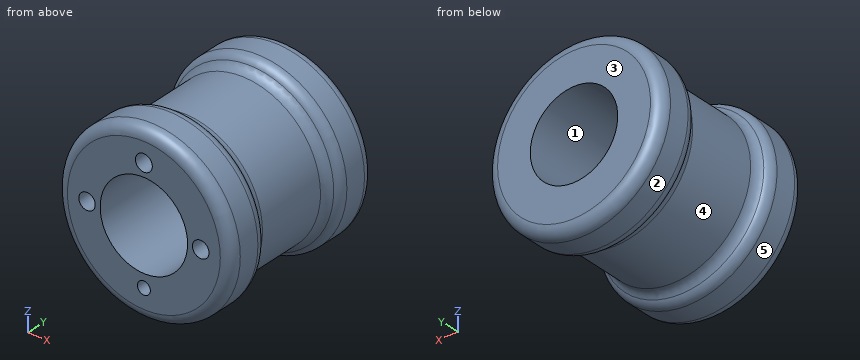
```python
from build123d import *

# Parameters (mm, degrees)
F0_R          = 12.7
F0_R_2        = 6.35
F1_DEPTH      = 25.4
F2_R          = 3.3757627259
F3_DEPTH      = 6.35
F4_R          = 12.7
F4_R_2        = 11.1125
F5_DEPTH      = 12.7
F6_R          = 4.2817922897
F7_DEPTH      = 25.4
F8_R          = 1.2247027219
F8_R_2        = 1.2053090412
F8_R_3        = 0.9363200651
F8_R_4        = 1.1938
F9_DEPTH      = 3.175
F10_S7_R      = 11.1125
F10_T8_DEPTH  = 21
F10_S13_R     = 11.1125
F10_T14_DEPTH = 21
F11_R         = 1.6002


# Not quite as in the source:
# - a fillet or chamfer that OpenCascade refuses, or shapes differently, is made with other operations: its cross-section is extruded or revolved along the edge and cut away or added


with BuildPart() as f1:
    # F0 (on Front) → F1 (new body)
    with BuildSketch(Plane.XZ):
        Circle(F0_R)
        Circle(F0_R_2, mode=Mode.SUBTRACT)
    extrude(amount=F1_DEPTH)

    # F4 (on face) → F5 (cut)
    with BuildSketch(Plane.XZ.offset(6.35)):
        Circle(F4_R)
        Circle(F4_R_2, mode=Mode.SUBTRACT)
    extrude(amount=F5_DEPTH, mode=Mode.SUBTRACT)

    # F8 (on face) → F9 (cut)
    with BuildSketch(Plane.XZ.offset(25.4)):
        with Locations((0, 8.255)):
            Circle(F8_R)
        with Locations((8.255, 0)):
            Circle(F8_R_2)
        with Locations((0, -8.255)):
            Circle(F8_R_3)
        with Locations((-8.255, 0)):
            Circle(F8_R_4)
    extrude(amount=-F9_DEPTH, mode=Mode.SUBTRACT)

    # F10: fillet of radius 1.6002 on 4 edges, made by hand

    # F10_s1 → F10_t2 (revolve, cut)
    with BuildSketch(Plane.XY):
        with BuildLine():
            ThreePointArc((11.0998, -25.4), (12.2313122713, -24.9313122713), (12.7, -23.7998))
            Line((12.7, -23.7998), (12.7, -25.4))
            Line((12.7, -25.4), (11.0998, -25.4))
        make_face()
    revolve(axis=Axis((0, -25.4, 0), (0, -1, 0)), mode=Mode.SUBTRACT)


with BuildPart() as f3:
    # F2 (on Front) → F3 (new body)
    with BuildSketch(Plane.XZ):
        Circle(F2_R)
    extrude(amount=F3_DEPTH)

    # F6 (on face) → F7 (cut)
    with BuildSketch(Plane.XZ.offset(6.35)):
        Circle(F6_R)
    extrude(amount=-F7_DEPTH, mode=Mode.SUBTRACT)


with BuildPart() as f10_tool4:
    # F10_s5 → F10_t6 (revolve)
    with BuildSketch(Plane.XY):
        with BuildLine():
            ThreePointArc((11.0998, -19.05), (12.2313122713, -19.5186877287), (12.7, -20.6502))
            Line((12.7, -20.6502), (12.7, -19.05))
            Line((12.7, -19.05), (11.0998, -19.05))
        make_face()
    revolve(axis=Axis((0, -19.05, 0), (0, -1, 0)))

    # F10_s7 → F10_t8 (cut, symmetric)
    with BuildSketch(Plane.XZ.offset(20.4)):
        Circle(F10_S7_R)
    extrude(amount=F10_T8_DEPTH, both=True, mode=Mode.SUBTRACT)


with BuildPart() as f1_1:
    add(f1.part)

    # F10_t3: cut F10_tool4
    add(f10_tool4.part, mode=Mode.SUBTRACT)


with BuildPart() as f10_tool10:
    # F10_s11 → F10_t12 (revolve)
    with BuildSketch(Plane.XY):
        with BuildLine():
            ThreePointArc((12.7, -4.7498), (12.2313122713, -5.8813122713), (11.0998, -6.35))
            Line((11.0998, -6.35), (12.7, -6.35))
            Line((12.7, -6.35), (12.7, -4.7498))
        make_face()
    revolve(axis=Axis((0, -6.35, 0), (0, -1, 0)))

    # F10_s13 → F10_t14 (cut, symmetric)
    with BuildSketch(Plane.XZ.offset(5.5)):
        Circle(F10_S13_R)
    extrude(amount=F10_T14_DEPTH, both=True, mode=Mode.SUBTRACT)


with BuildPart() as f1_2:
    add(f1_1.part)

    # F10_t9: cut F10_tool10
    add(f10_tool10.part, mode=Mode.SUBTRACT)

    # F10_s15 → F10_t16 (revolve, cut)
    with BuildSketch(Plane.XY):
        with BuildLine():
            ThreePointArc((12.7, -1.6002), (12.2313122713, -0.4686877287), (11.0998, 0))
            Line((11.0998, 0), (12.7, 0))
            Line((12.7, 0), (12.7, -1.6002))
        make_face()
    revolve(axis=Axis((0, 0, 0), (0, -1, 0)), mode=Mode.SUBTRACT)

    # F11
    f11_edges = [f1_2.edges().sort_by_distance(p)[0] for p in [
        (-11.1125, -19.05005, 0),
        (-11.1125, -6.34995, 0),
    ]]
    fillet(f11_edges, radius=F11_R)


solid = f1_2.part
```
Source: CAD feature listing. Evaluate the final solid. Frame: model axes, mm. Face numbers are marked on the shaded views. A direction names the side the tool comes from. Give positions to 0.01 mm unless a question says otherwise; leave off trailing zeros. Use a Markdown table: item, result. Add a question column.
(1) Access query for the marked faces 4 and 5. Directions: +Z, -Z, +X, -X, +Y, -Y. A direction counts if a zero-diameter tool reaches every point of the face in a straight line with its end or side. Return the directions, or none.
(2) Ray query, line 1 (Z direction, x = 0, y = -23.75); line 2 (Z direction, x = 0, y = -9); line 3 (Y direction, x = -11.25, z = 1.25). Return the intervals inside material, ascending.
(3) First-contact query: pin 1 Ø2 at (y, z) = (-10, 4) entering from +X; pin 2 Ø6 at (x, y) = (-9.5, -10) entering from -Z; pin 3 Ø1.2 at (x, z) = (-8.5, 0) entering from -Y (3 decimals). Flat tips, straight axial feed; report the tip coordinate or a pass-through.
(4) Pull-direction query (Z, two-part tool) for the marked faces 1, 2 and 3; classes: +Z half, -Z half, draft (parallel to the pull), parting line (faces both ways), or undercut.
Checked values:
| question | item | result |
|---|---|---|
| 1 | face 4 | none |
| 1 | face 5 | +Y, -Y |
| 2 | line 1 | -12.7 to -9.19, -7.32 to -6.35, 6.35 to 7.03, 9.48 to 12.7 |
| 2 | line 2 | -11.11 to -6.35, 6.35 to 11.11 |
| 2 | line 3 | -25.38 to -18.67, -6.73 to -0.02 |
| 3 | pin 1 | x = 10.7 |
| 3 | pin 2 | z = -9.01 |
| 3 | pin 3 | y = -22.225 |
| 4 | face 1 | undercut |
| 4 | face 2 | parting line |
| 4 | face 3 | draft |
